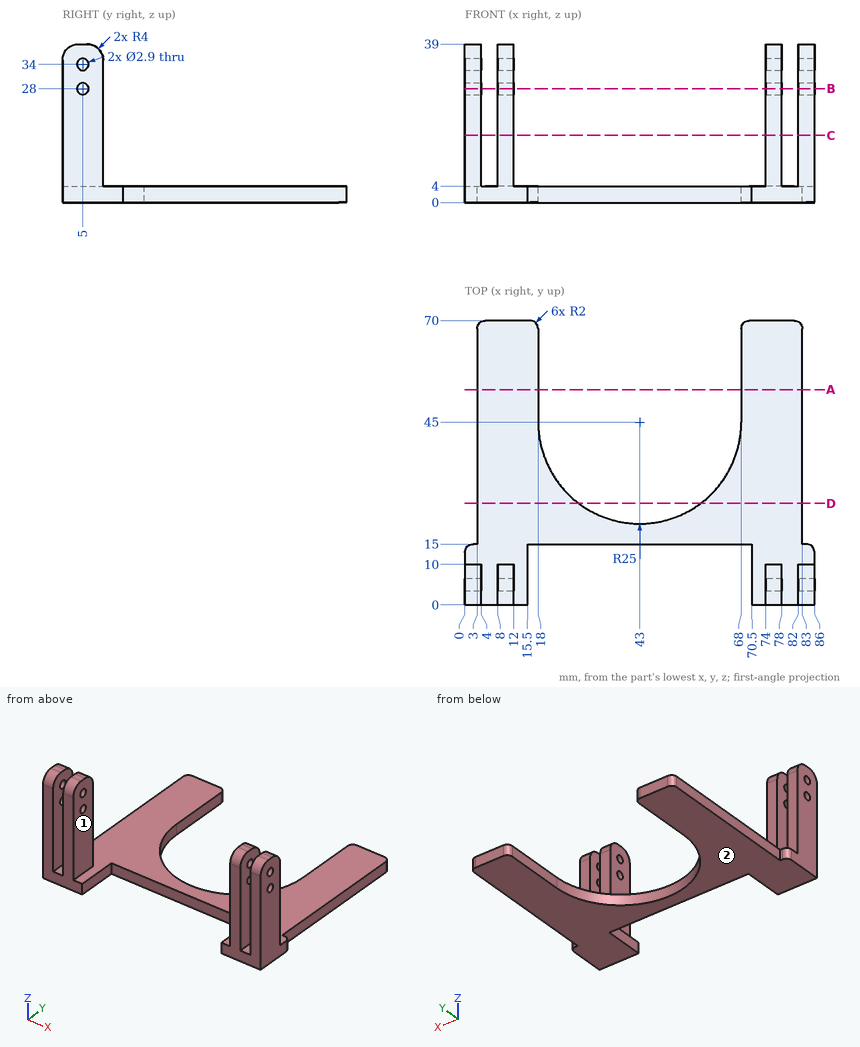
The drawing under review shows one solid part. Ordinate dimensions are in mm from its lowest x, y, z. A direction names the side the tool comes from. Give positions to 0.01 mm unless a question says otherwise; leave off trailing zeros. Write each loop counter-clockwise with the first axis right and the second up, starting at its lowest first coordinate (ties: lowest second). Pieces come first, ordered by that corner, then holes. Notation, with made-up numbers: (68, 39.25) - (89, 39.25) arc R17 cw to (89, 50.25) - close; hole circle Ø9 at (-37.75, -35). An arc over 180 degrees is marked (long way). Answer in a Markdown table with one row per item. Add a question column.
1. We need section C-C on z = 16.5. Write out the cut boundary in (x, y), then the cut area to 3 significant figures.
2. We need section B-B on z = 28. State how many separate pieces and enclosed holes the cut face has, then the cut area to 3 significant figures.
3. We need section A-A on y = 53. Write out the cut boundary in (x, z).
4. Insertion check: P1, Ø1.2, axis at x = 76, z = 15.5, coming from the +Y side; P2, Ø2, axis at y = 43.5, z = 2, coming from the +X side; P3, Ø1.2, axis at x = 49.5, z = 1, coming from the -Y side. Each pin has a flat end and moves straight along its axis. Give the tip position at first contact, or say it passes through.
5. Wall thickness on line 1 along Z through (x, y) = (75, 5); line 2 along Y through (x, z) = (83, 34); line 3 along X through (y, z) = (11.5, 3): over which ranges is each line inside the solid? List them lowest first. Write a range as [from, to].
6. We need section D-D on y = 25. Write out the cut boundary in (x, z).
7. Tool access review of the marked faces 1 and 2: name each direction out of +Z, -Z, +X, -X, +Y, -Y from which nothing blocks a thin tool from reaching the whole face with its end or side.
Ans:
| question | item | result |
|---|---|---|
| 1 | outline | (0, 0) - (4, 0) - (4, 10) - (0, 10) - close; (8, 0) - (12, 0) - (12, 10) - (8, 10) - close; (74, 0) - (78, 0) - (78, 10) - (74, 10) - close; (82, 0) - (86, 0) - (86, 10) - (82, 10) - close |
| 1 | area | 160 mm^2 |
| 2 | separate pieces | 8 |
| 2 | enclosed holes | 0 |
| 2 | area | 114 mm^2 |
| 3 | outline | (3, 0) - (18, 0) - (18, 4) - (3, 4) - close; (68, 0) - (83, 0) - (83, 4) - (68, 4) - close |
| 4 | P1 | stops at y = 10 |
| 4 | P2 | stops at x = 83 |
| 4 | P3 | stops at y = 15 |
| 5 | line 1 | z = [0, 26.55], [29.45, 32.55], [35.45, 39] |
| 5 | line 2 | y = [0, 3.55], [6.45, 10] |
| 5 | line 3 | x = [0, 15.5], [70.5, 86] |
| 6 | outline | (3, 0) - (28, 0) - (28, 4) - (3, 4) - close; (58, 0) - (83, 0) - (83, 4) - (58, 4) - close |
| 7 | face 1 | +Z, +Y, -Y |
| 7 | face 2 | -Z, +X, -X, +Y, -Y |
